```python
from build123d import *

# Parameters (mm, degrees)
SKETCH1_R                 = 23
BOSS_EXTRUDE1_DEPTH       = 5.5
SKETCH2_R                 = 4
CUT_EXTRUDE1_DEPTH        = 5.5
M3X0_5_TAPPED_HOLE1_D     = 2.5
M3X0_5_TAPPED_HOLE1_DEPTH = 6.5
M3X0_5_TAPPED_HOLE1_TIP   = 0.751075774
SKETCH6_R                 = 6
SKETCH6_R_2               = 4
BOSS_EXTRUDE2_DEPTH       = 1


with BuildPart() as part:
    # Sketch1 → Boss-Extrude1 (new body)
    with BuildSketch(Plane(origin=(0, 0, 0), x_dir=(1, 0, 0), z_dir=(0, 1, 0))):
        Circle(SKETCH1_R)
    extrude(amount=BOSS_EXTRUDE1_DEPTH)

    # Sketch2 → Cut-Extrude1 (cut)
    with BuildSketch(Plane(origin=(0, 5.5, 0), x_dir=(1, 0, 0), z_dir=(0, 1, 0))):
        Circle(SKETCH2_R)
    extrude(amount=-CUT_EXTRUDE1_DEPTH, mode=Mode.SUBTRACT)

    # M3x0.5 Tapped Hole1
    with Locations(Plane(origin=(0, 0, 0), x_dir=(-1, 0, 0), z_dir=(0, -1, 0))):
        with Locations((6.717514421, -6.717514421), (-7.5, 0), (0, 7.5), (7.5, 0), (0, -7.5), (-6.717514421, -6.717514421), (-6.717514421, 6.717514421), (6.717514421, 6.717514421)):
            Hole(M3X0_5_TAPPED_HOLE1_D / 2, depth=M3X0_5_TAPPED_HOLE1_DEPTH)
            with Locations((0, 0, -(M3X0_5_TAPPED_HOLE1_DEPTH + M3X0_5_TAPPED_HOLE1_TIP / 2))):  # 118° drill point
                Cone(0, M3X0_5_TAPPED_HOLE1_D / 2, M3X0_5_TAPPED_HOLE1_TIP, mode=Mode.SUBTRACT)

    # Sketch6 → Boss-Extrude2 (add)
    with BuildSketch(Plane.XZ):
        Circle(SKETCH6_R)
        Circle(SKETCH6_R_2, mode=Mode.SUBTRACT)
    extrude(amount=BOSS_EXTRUDE2_DEPTH)


solid = part.part
```
Here's how the part is built. I have some questions about the finished solid (model axes, mm). Give positions to 0.01 mm unless a question says otherwise; leave off trailing zeros. Loops run counter-clockwise (first coordinate to the right, second up) from the corner with the lowest first, then second, coordinate; pieces in that order, holes last. Notation, with made-up numbers: M 49,-9.75 L 61,-9.75 A26 cw 61,29.25 Z; hole C -10,51.25 d5. An arc over 180 degrees is marked long. Return JSON: item names as keys, results as strings.
Item 1: Please list where these lines run through material, in increasing order: line 1 (Z direction, x = 0, y = 4.35); line 2 (Z direction, x = -7.5, y = 2.3); line 3 (X direction, y = 1.75, z = 6).
A:
{"line 1": "z = -23 to -8.75, -6.25 to -4, 4 to 6.25, 8.75 to 23", "line 2": "z = -21.74 to -7.69, -5.74 to -1.25, 1.25 to 5.74, 7.69 to 21.74", "line 3": "x = -22.2 to -7.74, -5.69 to 5.69, 7.74 to 22.2"}
Item 2: Imagine slicing it at A-A on x = 0. List the corners of the cut face in (y, z) for me.
A:
{"outline": "M -1,-6 L 0,-6 L 0,-6.25 L 5.5,-6.25 L 5.5,-4 L -1,-4 Z; M -1,4 L 5.5,4 L 5.5,6.25 L 0,6.25 L 0,6 L -1,6 Z; M 0,-23 L 5.5,-23 L 5.5,-8.75 L 0,-8.75 Z; M 0,8.75 L 5.5,8.75 L 5.5,23 L 0,23 Z"}
Item 3: Thinking about a two-plate mould opening in Z: for faces 1 (the flat face through (5, 0, 5)), 2 (the cylindrical face through (-5.994, -0.493, 0.264)), 3 (the cylindrical face through (-7.966, 2.788, -6.772)), 4 (the cylindrical face through (-8.75, 2.79, -0.05)), which applies, released by +Z, released by -Z, zero draft, split by the parting line, or undercut?
A:
{"face 1": "zero draft", "face 2": "split by the parting line", "face 3": "undercut", "face 4": "undercut"}
Item 4: I'm going to push flat-ended pins straight in: pin 1 Ø8 at (x, z) = (10.5, 2) entering from -Y; pin 2 Ø3 at (y, z) = (1, 13.5) entering from +X. Where does each tip first touch, or does it pass through?
A:
{"pin 1": "stops at y = 0", "pin 2": "stops at x = 19.62"}
Item 5: Imagine slicing it at D-D on x = 19. List the corners of the cut face in (y, z) for me.
A:
{"outline": "M 0,-12.96 L 5.5,-12.96 L 5.5,12.96 L 0,12.96 Z"}
Item 6: Imagine slicing it at B-B on z = 0. List the corners of the cut face in (x, y) for me, then the cut area to 4 significant figures.
A:
{"outline": "M -23,0 L -8.75,0 L -8.75,5.5 L -23,5.5 Z; M -6.25,0 L -6,0 L -6,-1 L -4,-1 L -4,5.5 L -6.25,5.5 Z; M 4,-1 L 6,-1 L 6,0 L 6.25,0 L 6.25,5.5 L 4,5.5 Z; M 8.75,0 L 23,0 L 23,5.5 L 8.75,5.5 Z", "area": "185.5 mm^2"}
Item 7: Imagine slicing it at C-C on y = 4.25. State how many separate pieces and enclosed holes the cut face has, then the cut area to 3 significant figures.
A:
{"separate pieces": "1", "enclosed holes": "9", "area": "1,570 mm^2"}
